Check sheet for the modelled part. Datum: model origin and axes. Units: mm. Give positions to 0.01 mm unless a question says otherwise; leave off trailing zeros. Write each loop counter-clockwise with the first axis right and the second up, starting at its lowest first coordinate (ties: lowest second). Pieces come first, ordered by that corner, then holes. Notation, with made-up numbers: (59.25, -23.75) -> (72.25, -23.75) arc R30 ccw to (72.25, 3.25) -> close; hole circle Ø3 at (-38.5, 52). An arc over 180 degrees is marked (long way). Answer as a JSON object with one key per item and string values.
from build123d import *

# Parameters (mm, degrees)
SKETCH1_W          = 234.95
SKETCH1_H          = 86.36
BASE_FLANGE1_DEPTH = 3.175
SKETCH11_R         = 6.35
CUT_EXTRUDE3_DEPTH = 126.199715056
SKETCH12_R         = 3.81
CUT_EXTRUDE4_DEPTH = 126.199715056
SKETCH13_R         = 11.43
CUT_EXTRUDE5_DEPTH = 126.199715056
SKETCH14_R         = 3.81
CUT_EXTRUDE6_DEPTH = 126.199715056


# Sheet-metal steps are written as plain solids
with BuildPart() as part:
    # Sketch1 → Base-Flange1 (new body)
    with BuildSketch(Plane.XY):
        Rectangle(SKETCH1_W, SKETCH1_H)
    extrude(amount=-BASE_FLANGE1_DEPTH)

    # Sketch11 → Cut-Extrude3 (cut, through all)
    with BuildSketch(Plane.XY):
        with Locations((41.275, 17.78)):
            Circle(SKETCH11_R)
        with Locations((66.675, 17.78)):
            Circle(SKETCH11_R)
        with Locations((92.075, 17.78)):
            Circle(SKETCH11_R)
    extrude(amount=-CUT_EXTRUDE3_DEPTH, mode=Mode.SUBTRACT)

    # Sketch12 → Cut-Extrude4 (cut, through all)
    with BuildSketch(Plane.XY):
        with Locations((92.075, -16.51)):
            Circle(SKETCH12_R)
        with Locations((53.975, -16.51)):
            Circle(SKETCH12_R)
        with Locations((15.875, -16.51)):
            Circle(SKETCH12_R)
        with BuildLine():
            Line((8.763, -15.621), (8.763, -17.399))
            ThreePointArc((8.763, -17.399), (7.874, -18.288), (6.985, -17.399))
            Line((6.985, -17.399), (6.985, -15.621))
            ThreePointArc((6.985, -15.621), (7.874, -14.732), (8.763, -15.621))
        make_face()
        with BuildLine():
            Line((46.863, -15.621), (46.863, -17.399))
            ThreePointArc((46.863, -17.399), (45.974, -18.288), (45.085, -17.399))
            Line((45.085, -17.399), (45.085, -15.621))
            ThreePointArc((45.085, -15.621), (45.974, -14.732), (46.863, -15.621))
        make_face()
        with BuildLine():
            Line((84.963, -15.621), (84.963, -17.399))
            ThreePointArc((84.963, -17.399), (84.074, -18.288), (83.185, -17.399))
            Line((83.185, -17.399), (83.185, -15.621))
            ThreePointArc((83.185, -15.621), (84.074, -14.732), (84.963, -15.621))
        make_face()
    extrude(amount=-CUT_EXTRUDE4_DEPTH, mode=Mode.SUBTRACT)

    # Sketch13 → Cut-Extrude5 (cut, through all)
    with BuildSketch(Plane.XY):
        with Locations((-59.055, 12.192)):
            Circle(SKETCH13_R)
    extrude(amount=-CUT_EXTRUDE5_DEPTH, mode=Mode.SUBTRACT)

    # Sketch14 → Cut-Extrude6 (cut, through all)
    with BuildSketch(Plane.XY):
        with Locations((15.875, 17.78)):
            Circle(SKETCH14_R)
        with BuildLine():
            Line((8.763, 18.669), (8.763, 16.891))
            ThreePointArc((8.763, 16.891), (7.874, 16.002), (6.985, 16.891))
            Line((6.985, 16.891), (6.985, 18.669))
            ThreePointArc((6.985, 18.669), (7.874, 19.558), (8.763, 18.669))
        make_face()
    extrude(amount=-CUT_EXTRUDE6_DEPTH, mode=Mode.SUBTRACT)


solid = part.part
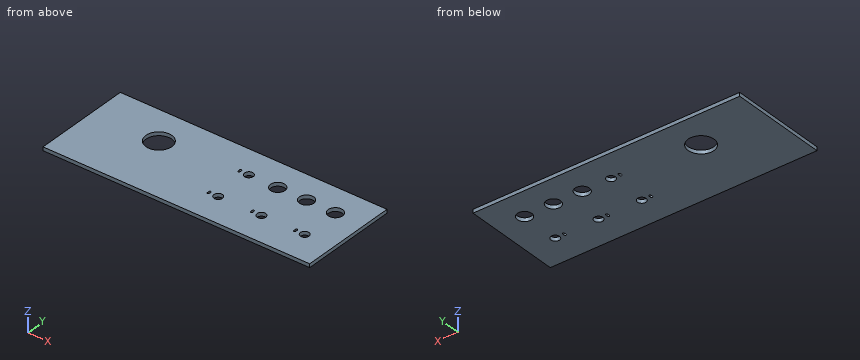
1. Sectioned sample at A-A, the plane x = 15.5. Enter the section's corners in (y, z) (1 decimal).
Determined:
{"outline": "(-43.2, -3.2) -> (-20.3, -3.2) -> (-20.3, 0) -> (-43.2, 0) -> close; (-12.7, -3.2) -> (14, -3.2) -> (14, 0) -> (-12.7, 0) -> close; (21.6, -3.2) -> (43.2, -3.2) -> (43.2, 0) -> (21.6, 0) -> close"}
2. Scan lines: L1, parallel to Y at x = 13.5, z = -0.5; L2, parallel to Y at x = 93, z = -2.85; L3, parallel to X at y = -14, z = -2.05 (3 decimals). Record each from-to range of solid material in increasing order. Write a range as [from, to].
Determined:
{"L1": "[-43.18, -19.49], [-13.53, 14.8], [20.76, 43.18]", "L2": "[-43.18, -20.21], [-12.81, 11.5], [24.06, 43.18]", "L3": "[-117.475, 13.009], [18.741, 51.109], [56.841, 89.209], [94.941, 117.475]"}
3. Sectioned sample at B-B, the plane z = -1.5. State how many separate pieces and enclosed holes the cut face has, plus the area to 3 significant figures.
Determined:
{"separate pieces": "1", "enclosed holes": "12", "area": "19,300 mm^2"}
